```python
from build123d import *

# Parameters (mm, degrees)
BASE_FLANGE1_DEPTH    = 0.7
EDGE_FLANGE1_DEPTH    = 35
EDGE_FLANGE2_DEPTH    = 35
BREAK_CORNER1_START   = -1.4366
BREAK_CORNER1_DEPTH   = 0.7
BREAK_CORNER1_START_2 = -0.7
BREAK_CORNER1_2_DEPTH = 0.7
BREAK_CORNER1_START_3 = -51.4366
BREAK_CORNER1_3_DEPTH = 0.7


# Read off the part's stored shape, not the designer's step: Break-Corner1
# Sheet-metal steps are written as plain solids
with BuildPart() as part:
    # Sketch1 → Base-Flange1 (new body)
    with BuildSketch(Plane(origin=(0, 0, 0), x_dir=(0, 0, -1), z_dir=(1, 0, 0))):
        Polygon((0, 0), (50, 50), (50, 0), align=None)
    extrude(amount=-BASE_FLANGE1_DEPTH)

    # Edge-Flange1 section (across the edge) → Edge-Flange1 (add)
    with BuildSketch(Plane(origin=(-0.7, 50, -50.7366), x_dir=(0, 0, 1), z_dir=(0, -1, 0))):
        with BuildLine():
            Line((-0.7, 0.7366), (-0.7, 10))
            Line((-0.7, 10), (0, 10))
            Line((0, 10), (0, 0.7366))
            ThreePointArc((0, 0.7366), (0.215745145, 0.215745145), (0.7366, 0))
            Line((0.7366, 0), (0.7366, -0.7))
            ThreePointArc((0.7366, -0.7), (-0.279229602, -0.279229602), (-0.7, 0.7366))
        make_face()
    extrude(amount=EDGE_FLANGE1_DEPTH)

    # Edge-Flange2 section (across the edge) → Edge-Flange2 (add)
    with BuildSketch(Plane(origin=(-0.7, -0.7366, -35), x_dir=(0, 1, 0), z_dir=(0, 0, 1))):
        with BuildLine():
            Line((-0.7, 0.7366), (-0.7, 10.1366))
            Line((-0.7, 10.1366), (0, 10.1366))
            Line((0, 10.1366), (0, 0.7366))
            ThreePointArc((0, 0.7366), (0.215745145, 0.215745145), (0.7366, 0))
            Line((0.7366, 0), (0.7366, -0.7))
            ThreePointArc((0.7366, -0.7), (-0.279229602, -0.279229602), (-0.7, 0.7366))
        make_face()
    extrude(amount=EDGE_FLANGE2_DEPTH)

    # Break-Corner1 outline → Break-Corner1 (cut)
    with BuildSketch(Plane(origin=(0, 0, 0), x_dir=(1, 0, 0), z_dir=(0, 1, 0)).offset(BREAK_CORNER1_START)):
        with BuildLine():
            ThreePointArc((-8.3366, 0), (-10.104366953, 0.732233047), (-10.8366, 2.5))
            Line((-10.8366, 2.5), (-10.8366, 0))
            Line((-10.8366, 0), (-8.3366, 0))
        make_face()
        with BuildLine():
            ThreePointArc((-10.8366, 32.5), (-10.104366953, 34.267766953), (-8.3366, 35))
            Line((-8.3366, 35), (-10.8366, 35))
            Line((-10.8366, 35), (-10.8366, 32.5))
        make_face()
    extrude(amount=BREAK_CORNER1_DEPTH, mode=Mode.SUBTRACT)

    # Break-Corner1 2 outline → Break-Corner1 2 (cut)
    with BuildSketch(Plane.YZ.offset(BREAK_CORNER1_START_2)):
        with BuildLine():
            ThreePointArc((2.5, -50), (0.732233047, -49.267766953), (0, -47.5))
            Line((0, -47.5), (0, -50))
            Line((0, -50), (2.5, -50))
        make_face()
    extrude(amount=BREAK_CORNER1_2_DEPTH, mode=Mode.SUBTRACT)

    # Break-Corner1 3 outline → Break-Corner1 3 (cut)
    with BuildSketch(Plane.XY.offset(BREAK_CORNER1_START_3)):
        with BuildLine():
            Line((-10.7, 50), (-10.7, 47.5))
            ThreePointArc((-10.7, 47.5), (-9.967766953, 49.267766953), (-8.2, 50))
            Line((-8.2, 50), (-10.7, 50))
        make_face()
        with BuildLine():
            ThreePointArc((-8.2, 15), (-9.967766953, 15.732233047), (-10.7, 17.5))
            Line((-10.7, 17.5), (-10.7, 15))
            Line((-10.7, 15), (-8.2, 15))
        make_face()
    extrude(amount=BREAK_CORNER1_3_DEPTH, mode=Mode.SUBTRACT)


solid = part.part
```
Work out the finished part from the listing and answer in its coordinate system (mm). A direction names the side the tool comes from. Coordinates: 2 decimals unless noted, no trailing zeros. Order: outer loops, then holes, each group sorted by start corner. A loop starts at its lowest first (then second) coordinate and runs counter-clockwise, first axis right, second up. Notation, with made-up numbers: (-14.5, 54.5) - (29.5, 54.5) arc R22 ccw to (29.5, 64.5) - close; hole circle Ø7 at (-19.5, 35.25). An arc over 180 degrees is marked (long way). Answer as a JSON object with one key per item and string values.
1. Find section D-D on x = -9.75. Determine the outline of the cut face in (y, z).
Output values:
{"outline": "(-1.44, -34.56) - (-0.74, -34.56) - (-0.74, -0.44) - (-1.44, -0.44) - close; (15.54, -51.44) - (49.46, -51.44) - (49.46, -50.74) - (15.54, -50.74) - close"}
2. Consider line 1 (X direction, y = 19, z = -21); line 2 (Y direction, x = -10.25, z = -30); line 3 (Z direction, x = -2.5, y = 15.5). Determine where each line is inside the solid, lowest interval first.
Output values:
{"line 1": "x = -0.7 to 0", "line 2": "y = -1.44 to -0.74", "line 3": "z = -51.44 to -50.74"}
3. Find section A-A on x = -4.75. Determine the outline of the cut face in (y, z).
Output values:
{"outline": "(-1.44, -35) - (-0.74, -35) - (-0.74, 0) - (-1.44, 0) - close; (15, -51.44) - (50, -51.44) - (50, -50.74) - (15, -50.74) - close"}
4. A tool of negligible diameter and unlimited length cuts with its end or side. For faces 1 (the face through (-0.7, 14, -36)), 2 (the face through (-6, -1.437, -18)), 3 (the face through (-6, -0.737, -18)), 4 (the face through (-6, 33, -50.737)), 5 (the face through (-4, -1, -35)), from which of +Z, -Z, +X, -X, +Y, -Y can it reach the whole face along a straight path? Write none if from no direction.
Output values:
{"face 1": "+Z, -X, +Y", "face 2": "+Z, -Z, +X, -X, -Y", "face 3": "+Z, -Z, -X, +Y", "face 4": "+Z, -X, +Y, -Y", "face 5": "-Z, +X, -X, -Y"}
5. Each of these flat-tipped pins is pushed along its axis until it touches: P1, Ø3, axis at x = -5.5, y = 34, coming from the +Z side; P2, Ø12, axis at y = 40.5, z = -44, coming from the -X side; P3, Ø0.6, axis at y = 33.5, z = -51, coming from the -X side. Where does it stop, or does it pass through?
Output values:
{"P1": "stops at z = -50.74", "P2": "stops at x = -0.7", "P3": "stops at x = -10.7"}
6. Find section C-C on y = 41. Determine the outline of the cut face in (x, z).
Output values:
{"outline": "(-10.7, -51.44) - (-1.44, -51.44) arc R1.44 ccw to (0, -50) - (0, -41) - (-0.7, -41) - (-0.7, -50) arc R0.74 cw to (-1.44, -50.74) - (-10.7, -50.74) - close"}
7. Find section B-B on z = -10. Determine the outline of the cut face in (x, y).
Output values:
{"outline": "(-10.84, -1.44) - (-1.44, -1.44) arc R1.44 ccw to (0, 0) - (0, 10) - (-0.7, 10) - (-0.7, 0) arc R0.74 cw to (-1.44, -0.74) - (-10.84, -0.74) - close"}
